Geometry check sheet. Reference: the model listing, model coordinates, mm. Face numbers are marked on the shaded views. Give positions to 0.01 mm unless a question says otherwise; leave off trailing zeros. Write each loop counter-clockwise with the first axis right and the second up, starting at its lowest first coordinate (ties: lowest second). Pieces come first, ordered by that corner, then holes. Notation, with made-up numbers: (60.25, 12.5) - (64.25, 12.5) arc R23 cw to (64.25, 51.5) - close; hole circle Ø7 at (-1, -4). An arc over 180 degrees is marked (long way). One line per question, with ' | ' between items. Start each with the question number.
Q1. Thickness scan on L1, parallel to Z at x = 503.5, y = 17; L2, parallel to Y at x = 0, z = 12.5; L3, parallel to X at y = 13, z = 0. Record the ranges inside material, lowest first. Write a range as [from, to].
Q2. Section check D-D on x = 130.5. Record the boundary of the cut face in (y, z).
Q3. Release check for a two-part mould opening along X. For the marked faces 1, 2 and 3 record: +X half, -X half, draft (parallel to the pull), parting line (faces both ways), or undercut.
Q4. Section check A-A on z = -9. Record the boundary of the cut face in (x, y).
Q5. Section check C-C on x = 395.5. Record the boundary of the cut face in (y, z).
Q6. Gauge pin test, flat ends, axial feed: P1, Ø6, axis at y = 33.5, z = -10, coming from the -X side; P2, Ø4, axis at y = 12, z = 17.5, coming from the +X side. Record the tip position at first contact, or that the pin passes through.
Q7. Section check B-B on y = 0. Record the boundary of the cut face in (x, z).
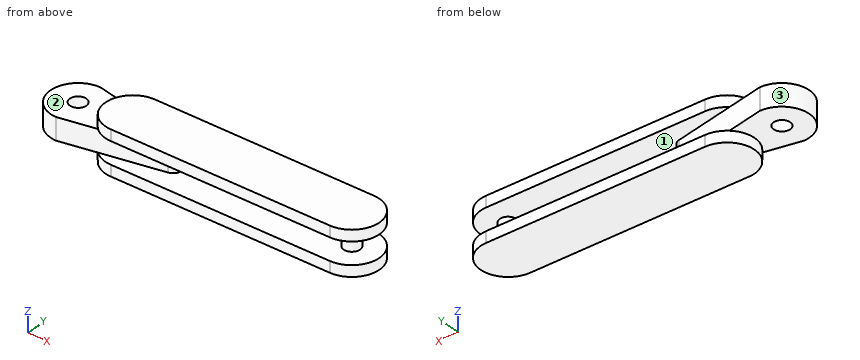
```python
from build123d import *

# Parameters (mm, degrees)
BOSS_EXTRUDE2_DEPTH = 40
CUT_EXTRUDE2_DEPTH  = 20
CUT_EXTRUDE3_START  = -20
CUT_EXTRUDE3_DEPTH  = 20
SKETCH9_R           = 15
CUT_EXTRUDE5_DEPTH  = 40
CUT_EXTRUDE6_DEPTH  = 20
SKETCH13_R          = 15
BOSS_EXTRUDE4_DEPTH = 60
SKETCH11_R          = 15
BOSS_EXTRUDE3_DEPTH = 80


with BuildPart() as part:
    # Sketch4 → Boss-Extrude2 (new, symmetric)
    with BuildSketch(Plane.XY):
        with BuildLine():
            Line((-250, 50), (250, 50))
            ThreePointArc((250, 50), (300, 0), (250, -50))
            Line((250, -50), (-250, -50))
            ThreePointArc((-250, -50), (-300, 0), (-250, 50))
        make_face()
    extrude(amount=BOSS_EXTRUDE2_DEPTH, both=True)

    # Sketch5 → Cut-Extrude2 (cut)
    with BuildSketch(Plane.XY.offset(40)):
        with BuildLine():
            Line((-150, 50), (-250, 50))
            ThreePointArc((-250, 50), (-300, 0), (-250, -50))
            Line((-250, -50), (-150, -50))
            ThreePointArc((-150, -50), (-200, 0), (-150, 50))
        make_face()
    extrude(amount=-CUT_EXTRUDE2_DEPTH, mode=Mode.SUBTRACT)

    # Sketch6 → Cut-Extrude3 (cut)
    with BuildSketch(Plane(origin=(0, 0, -40), x_dir=(-1, 0, 0), z_dir=(0, 0, -1)).offset(CUT_EXTRUDE3_START)):
        with BuildLine():
            Line((150, 50), (250, 50))
            ThreePointArc((250, 50), (300, 0), (250, -50))
            Line((250, -50), (150, -50))
            ThreePointArc((150, -50), (200, 0), (150, 50))
        make_face()
    extrude(amount=CUT_EXTRUDE3_DEPTH, mode=Mode.SUBTRACT)

    # Sketch9 → Cut-Extrude5 (cut)
    with BuildSketch(Plane.XY.offset(20)):
        with Locations((-250, 0)):
            Circle(SKETCH9_R)
    extrude(amount=-CUT_EXTRUDE5_DEPTH, mode=Mode.SUBTRACT)

    # Sketch10 → Cut-Extrude6 (cut, symmetric)
    with BuildSketch(Plane.XY):
        with BuildLine():
            Line((-250, 50), (-73.543550677, 14.708710135))
            ThreePointArc((-73.543550677, 14.708710135), (-61.485292704, 0), (-73.543550677, -14.708710135))
            Line((-73.543550677, -14.708710135), (-250, -50))
            Line((-250, -50), (250, -50))
            ThreePointArc((250, -50), (300, 0), (250, 50))
            Line((250, 50), (-250, 50))
        make_face()
    extrude(amount=CUT_EXTRUDE6_DEPTH, both=True, mode=Mode.SUBTRACT)

    # Sketch13 → Boss-Extrude4 (add)
    with BuildSketch(Plane.XY.offset(40)):
        with Locations((250, 0)):
            Circle(SKETCH13_R)
    extrude(amount=-BOSS_EXTRUDE4_DEPTH)

    # Sketch11 → Boss-Extrude3 (add)
    with BuildSketch(Plane.XY.offset(40)):
        with Locations((250, 0)):
            Circle(SKETCH11_R)
    extrude(amount=-BOSS_EXTRUDE3_DEPTH)


with BuildPart() as part_1:
    # Body-Move/Copy1: moved
    add(part.part.moved(Location((250, 0, 0))))


solid = part_1.part
```
Working result:
1) L1: z = [-40, -20], [20, 40] | L2: y = [-50, -15], [15, 50] | L3: x = [-48.28, -7.48], [7.48, 181], [492.52, 507.48]
2) outline: (-50, -40) - (50, -40) - (50, -20) - (23.9, -20) - (23.9, 20) - (50, 20) - (50, 40) - (-50, 40) - (-50, 20) - (-23.9, 20) - (-23.9, -20) - (-50, -20) - close
3) face 1: undercut | face 2: draft | face 3: -X half
4) outline: (0, -50) - (176.46, -14.71) arc R15 ccw to (176.46, 14.71) - (0, 50) arc R50 ccw to start; circle Ø30 at (500, 0); hole circle Ø30 at (0, 0)
5) outline: (-50, -40) - (50, -40) - (50, -20) - (-50, -20) - close; (-50, 20) - (50, 20) - (50, 40) - (-50, 40) - close
6) P1: stops at x = -39.62 | P2: stops at x = 511.18
7) outline: (-50, -20) - (-15, -20) - (-15, 20) - (-50, 20) - close; (15, -20) - (50, -20) - (50, -40) - (550, -40) - (550, -20) - (515, -20) - (515, 20) - (550, 20) - (550, 40) - (50, 40) - (50, 20) - (15, 20) - close; hole (188.51, -20) - (485, -20) - (485, 20) - (188.51, 20) - close
